Work out the finished part from the listing and answer in its coordinate system (mm). A direction names the side the tool comes from. Coordinates: 2 decimals unless noted, no trailing zeros. Write each loop counter-clockwise with the first axis right and the second up, starting at its lowest first coordinate (ties: lowest second). Pieces come first, ordered by that corner, then holes. Notation, with made-up numbers: (31, 68) - (48, 68) arc R32 cw to (48, 100) - close; hole circle Ø5 at (-10.5, 85). An arc over 180 degrees is marked (long way). One line per item, written item: value.
```python
from build123d import *

# Parameters (mm, degrees)
SKETCH1_R                                      = 2.5
BOSS_EXTRUDE1_DEPTH                            = 25
CUT_EXTRUDE3_START                             = -5
SKETCH6_R                                      = 2
CUT_EXTRUDE3_DEPTH                             = 64.373971656
SKETCH7_R                                      = 1
CUT_EXTRUDE4_DEPTH                             = 69.373971824
FILLET1_R                                      = 10
CSK_FOR_M2_FLAT_HEAD_MACHINE_SCREW1_AT_2_COUNT = 2
CSK_FOR_M2_FLAT_HEAD_MACHINE_SCREW1_AT_2_PITCH = 85.586213843
CSK_FOR_M2_FLAT_HEAD_MACHINE_SCREW2_AT_2_COUNT = 2
CSK_FOR_M2_FLAT_HEAD_MACHINE_SCREW2_AT_2_PITCH = 85.586213843


with BuildPart() as part:
    # Sketch1 → Boss-Extrude1 (new body)
    with BuildSketch(Plane(origin=(0, 0, 0), x_dir=(1, 0, 0), z_dir=(0, 1, 0))):
        with BuildLine():
            Line((-45, 0), (-40, 0))
            ThreePointArc((-40, 0), (-36.565439333, 16.216308038), (-26.85156768, 29.647821389))
            ThreePointArc((-26.85156768, 29.647821389), (-20.075175272, 28.67032155), (-18.676061955, 35.372372126))
            ThreePointArc((-18.676061955, 35.372372126), (0, 40), (18.676061955, 35.372372126))
            ThreePointArc((18.676061955, 35.372372126), (20.075175272, 28.67032155), (26.85156768, 29.647821389))
            ThreePointArc((26.85156768, 29.647821389), (36.565439333, 16.216308038), (40, 0))
            Line((40, 0), (45, 0))
            ThreePointArc((45, 0), (0, 45), (-45, 0))
        make_face()
        with Locations(Location((22.943057454, 32.766081772, 0), (0, 0, 270))):
            Circle(SKETCH1_R, mode=Mode.SUBTRACT)
        with Locations(Location((-22.943057454, 32.766081772, 0), (0, 0, 270))):
            Circle(SKETCH1_R, mode=Mode.SUBTRACT)
    extrude(amount=BOSS_EXTRUDE1_DEPTH)

    # Sketch6 → Cut-Extrude3 (cut, through all)
    with BuildSketch(Plane.XY.offset(CUT_EXTRUDE3_START)):
        with Locations((-42.5, 20)):
            Circle(SKETCH6_R)
        with Locations((-42.5, 10)):
            Circle(SKETCH6_R)
        with Locations((42.5, 20)):
            Circle(SKETCH6_R)
        with Locations((42.5, 10)):
            Circle(SKETCH6_R)
    extrude(amount=-CUT_EXTRUDE3_DEPTH, mode=Mode.SUBTRACT)

    # Sketch7 → Cut-Extrude4 (cut, through all)
    with BuildSketch(Plane.XY):
        with Locations((-42.5, 20)):
            Circle(SKETCH7_R)
        with Locations((-42.5, 10)):
            Circle(SKETCH7_R)
        with Locations((42.5, 10)):
            Circle(SKETCH7_R)
        with Locations((42.5, 20)):
            Circle(SKETCH7_R)
    extrude(amount=-CUT_EXTRUDE4_DEPTH, mode=Mode.SUBTRACT)

    # Fillet1
    fillet1_edges = [part.edges().sort_by_distance(p)[0] for p in [
        (26.85156768, 12.5, -29.647821389),
        (18.676061955, 12.5, -35.372372126),
        (-18.676061955, 12.5, -35.372372126),
        (-26.85156768, 12.5, -29.647821389),
    ]]
    fillet(fillet1_edges, radius=FILLET1_R)

    # Sketch17 → CSK for M2 Flat Head Machine Screw1 (revolve, cut)
    with BuildSketch(Plane(origin=(-42.5, 20, -5), x_dir=(0, 1, 0), z_dir=(1, 0, 0))):
        Polygon((0, 0), (0, 5), (1.3, 5), (1.3, 0.9), (2.2, 0), align=None)
    csk_for_m2_flat_head_machine_screw1 = revolve(axis=Axis((-42.5, 20, -11.35), (0, 0, 1)), mode=Mode.SUBTRACT)

    # CSK for M2 Flat Head Machine Screw1 at 2: CSK for M2 Flat Head Machine Screw1 ×2
    with Locations(*[Vector(0.9931506043228763, -0.11684124756739721, 0) * (i * CSK_FOR_M2_FLAT_HEAD_MACHINE_SCREW1_AT_2_PITCH) for i in range(1, CSK_FOR_M2_FLAT_HEAD_MACHINE_SCREW1_AT_2_COUNT)]):
        add(csk_for_m2_flat_head_machine_screw1, mode=Mode.SUBTRACT)

    # Sketch18 → CSK for M2 Flat Head Machine Screw2 (revolve, cut)
    with BuildSketch(Plane(origin=(42.5, 20, -5), x_dir=(0, 1, 0), z_dir=(1, 0, 0))):
        Polygon((0, 0), (0, 5), (1.3, 5), (1.3, 0.9), (2.2, 0), align=None)
    csk_for_m2_flat_head_machine_screw2 = revolve(axis=Axis((42.5, 20, -11.35), (0, 0, 1)), mode=Mode.SUBTRACT)

    # CSK for M2 Flat Head Machine Screw2 at 2: CSK for M2 Flat Head Machine Screw2 ×2
    with Locations(*[Vector(-0.9931506043228763, -0.11684124756739721, 0) * (i * CSK_FOR_M2_FLAT_HEAD_MACHINE_SCREW2_AT_2_PITCH) for i in range(1, CSK_FOR_M2_FLAT_HEAD_MACHINE_SCREW2_AT_2_COUNT)]):
        add(csk_for_m2_flat_head_machine_screw2, mode=Mode.SUBTRACT)


solid = part.part
```
Item 1: Given pin 1 (2 mm diameter, centred on x = 2, y = 9.5, fed in from +Z); pin 2 (1.5 mm diameter, centred on y = 5.5, z = -24.5, fed in from +X); pin 3 (12 mm diameter, centred on x = -10.5, y = 8.5, fed in from -Z), each flat-ended and moving along its own axis, determine where each tip first touches the part or whether it passes through.
Evaluation:
pin 1: stops at z = -39.89
pin 2: stops at x = 38.22
pin 3: stops at z = -44.77
Item 2: Consider probe 1 along Y at (x, z) = (-42.5, -8.5); probe 2 along X at (y, z) = (20, -1); probe 3 along X at (y, z) = (14.5, -33). Determine where each line is inside the solid, lowest interval first.
Evaluation:
probe 1: y = 0 to 8, 12 to 18, 22 to 25
probe 2: x = -44.99 to -43.8, -41.2 to -39.99, 39.99 to 41.2, 43.8 to 44.99
probe 3: x = -30.59 to -25.43, -20.45 to -17.55, 17.55 to 20.45, 25.43 to 30.59
Item 3: Section A-A, the plane z = -16.5 is taken. Determine the outline of the cut face in (x, y).
Evaluation:
outline: (-41.87, 0) - (-36.44, 0) - (-36.44, 25) - (-41.87, 25) - (-41.87, 21.9) arc R2 cw to (-41.87, 18.1) - (-41.87, 11.9) arc R2 cw to (-41.87, 8.1) - close; (36.44, 0) - (41.87, 0) - (41.87, 8.1) arc R2 cw to (41.87, 11.9) - (41.87, 18.1) arc R2 cw to (41.87, 21.9) - (41.87, 25) - (36.44, 25) - close
Item 4: Section C-C, the plane y = 20 is taken. Give the number of separate pieces and of enclosed holes in the cut face, then the cut area to 3 significant figures.
Evaluation:
separate pieces: 3
enclosed holes: 2
area: 631 mm2
Item 5: Section B-B, the plane x = 42.5 is taken. Determine the outline of the cut face in (y, z).
Evaluation:
outline: (0, -14.79) - (8, -14.79) - (8, -5) - (7.8, -5) - (8.7, -4.1) - (8.7, 0) - (0, 0) - close; (11.3, -4.1) - (12.2, -5) - (12, -5) - (12, -14.79) - (18, -14.79) - (18, -5) - (17.8, -5) - (18.7, -4.1) - (18.7, 0) - (11.3, 0) - close; (21.3, -4.1) - (22.2, -5) - (22, -5) - (22, -14.79) - (25, -14.79) - (25, 0) - (21.3, 0) - close
Item 6: Which of the six approach directions +Z, -Z, +X, -X, +Y, -Y give full straight-line access (tool end or side, diameter ignored) to faces 4 (the face through (-38.051, 12.325, -12.333)), 5 (the face through (-40.592, 20.601, -10.581)), 6 (the face through (42, 12, 0))?
Evaluation:
face 4: +Z, +Y, -Y
face 5: -Z
face 6: +Z, +X, -X, +Y, -Y
Item 7: Determine the mould class of faces 1 (the face through (20.036, 12.325, -28.698)), 2 (the face through (-40.592, 10.601, -10.581)), 3 (the face through (0, 25, -41)) for opening direction Y: +Y half, -Y half, draft (parallel to the pull), parting line (faces both ways), or undercut.
Evaluation:
face 1: draft
face 2: undercut
face 3: +Y half
